```python
from build123d import *

# Parameters (mm, degrees)
F0_R     = 25.4
F0_R_2   = 5.08
F0_W     = 3.81
F0_H     = 38.1
F1_DEPTH = 6.35
F2_R     = 2.54


with BuildPart() as f1:
    # F0 (on Top) → F1 (new body)
    with BuildSketch(Plane.XY):
        with Locations((-134.285456, 19.05)):
            Circle(F0_R)
        with BuildLine():
            ThreePointArc((-143.547478, 16.089377), (-142.087057, 14.306864), (-141.564401, 12.062535))
            ThreePointArc((-141.564401, 12.062535), (-151.201745, 9.818205), (-143.547478, 16.089377))
        make_face(mode=Mode.SUBTRACT)
        with Locations((-147.212275, 27.376856)):
            Circle(F0_R_2, mode=Mode.SUBTRACT)
        with Locations((-134.285456, 19.05)):
            Rectangle(F0_W, F0_H, mode=Mode.SUBTRACT)
    extrude(amount=F1_DEPTH)

    # F2
    f2_edges = [f1.edges().sort_by_distance(p)[0] for p in [
        (-159.685456, 19.05, 6.35),
        (-159.685456, 19.05, 0),
    ]]
    fillet(f2_edges, radius=F2_R)


solid = f1.part
```
The model under review builds one solid part; all positions refer to its coordinate system, in mm. A direction names the side the tool comes from. Coordinates: 2 decimals unless noted, no trailing zeros. Order: outer loops, then holes, each group sorted by start corner. A loop starts at its lowest first (then second) coordinate and runs counter-clockwise, first axis right, second up. Notation, with made-up numbers: (14.25, -14) -> (46.25, -14) arc R11 cw to (46.25, 0) -> close; hole circle Ø6 at (16, -6). An arc over 180 degrees is marked (long way). Answer in a Markdown table with one row per item. Add a question column.
Item 1: To check wall thickness, follow probe 1 along X at (y, z) = (7.5, 1); probe 2 along X at (y, z) = (28, 4.75); probe 3 along Y at (x, z) = (-148.5, 5.5). State the ranges of each line that lie inside material, in increasing order.
Item 2: Mouldability with a two-part tool opening along Y and no side actions: class faces 3 (the flat face through (-134, 38.1, 3)), 4 (the flat face through (-130, 19, 6.35)), 5 (the cylindrical face through (-110.06, 26.68, 3.17)) as +Y half, -Y half, draft (parallel to the pull), parting line (faces both ways), or undercut.
Item 3: We need section C-C on y = 28. Give the number of separate pieces and of enclosed holes in the cut face, plus the area to 3 significant figures.
Item 4: We need section A-A on y = 19.05. Write out the cut boundary in (x, z), plus the area to 3 significant figures.
Item 5: We need section B-B on z = 1.5. Write out the cut boundary in (x, y).
Item 6: Clearance check with flat-ended pins moving along their axes: pin 1 (1.5 mm diameter, centred on y = 10, z = 1, fed in from -X); pin 2 (1.1 mm diameter, centred on x = -135, z = 3.5, fed in from -Y); pin 3 (3 mm diameter, centred on x = -133.5, z = 4, fed in from +Y). State where each tip first meets the part, or that it passes through.
Item 7: Machinability: for faces 1 (the flat face through (-130, 19, 0)), 2 (the flat face through (-134, 0, 3)), which of the approach directions +Z, -Z, +X, -X, +Y, -Y give a long, thin tool a straight path to every point of the face, cutting with its end or side? Answer none if there is none.
Final values:
| question | item | result |
|---|---|---|
| 1 | probe 1 | x = -156.32 to -148.88, -144.41 to -136.19, -132.38 to -112.25 |
| 1 | probe 2 | x = -157.86 to -152.25, -142.17 to -136.19, -132.38 to -110.71 |
| 1 | probe 3 | y = -1.22 to 7.33, 16.79 to 22.46, 32.29 to 39.32 |
| 2 | face 3 | undercut |
| 2 | face 4 | draft |
| 2 | face 5 | parting line |
| 3 | separate pieces | 3 |
| 3 | enclosed holes | 0 |
| 3 | area | 208 mm2 |
| 4 | outline | (-159.69, 2.54) arc R2.54 ccw to (-157.15, 0) -> (-136.19, 0) -> (-136.19, 6.35) -> (-157.15, 6.35) arc R2.54 ccw to (-159.69, 3.81) -> close; (-132.38, 0) -> (-111.43, 0) arc R2.54 ccw to (-108.89, 2.54) -> (-108.89, 3.81) arc R2.54 ccw to (-111.43, 6.35) -> (-132.38, 6.35) -> close |
| 4 | area | 293 mm2 |
| 5 | outline | circle Ø50.35 at (-134.29, 19.05); hole circle Ø10.16 at (-147.21, 27.38); hole (-143.55, 16.09) arc R5.08 ccw (long way) to (-141.56, 12.06) arc R5.08 ccw to start; hole (-136.19, 0) -> (-132.38, 0) -> (-132.38, 38.1) -> (-136.19, 38.1) -> close |
| 6 | pin 1 | stops at x = -157.99 |
| 6 | pin 2 | stops at y = -6.35 |
| 6 | pin 3 | stops at y = 44.45 |
| 7 | face 1 | -Z, +X, -X, +Y, -Y |
| 7 | face 2 | +Z, -Z |
